The listing builds one solid part. Answer for the finished solid, in the listing's coordinates (mm). Face numbers are marked on the shaded views. Coordinates: 2 decimals unless noted, no trailing zeros. Answer in a Markdown table with one row per item.
```python
from build123d import *

# Parameters (mm, degrees)
F0_W      = 71.4375
F0_H      = 142.875
F1_DEPTH  = 6.35
F3_DEPTH  = 4.7625
F5_DEPTH  = 3.175
F6_R      = 3.175
F8_D      = 1.984375
F9_R      = 1.984375
F9_R_2    = 0.9921875
F10_DEPTH = 1.5875


with BuildPart() as f1:
    # F0 (on Top) → F1 (new body)
    with BuildSketch(Plane.XY):
        with BuildLine():
            Line((-40.084375, 71.4375), (-40.084375, 0))
            Line((-40.084375, 0), (-40.084375, -71.4375))
            ThreePointArc((-40.084375, -71.4375), (-39.1544390303, -73.6825640303), (-36.909375, -74.6125))
            Line((-36.909375, -74.6125), (36.909375, -74.6125))
            ThreePointArc((36.909375, -74.6125), (39.1544390303, -73.6825640303), (40.084375, -71.4375))
            Line((40.084375, -71.4375), (40.084375, 71.4375))
            ThreePointArc((40.084375, 71.4375), (39.1544390303, 73.6825640303), (36.909375, 74.6125))
            Line((36.909375, 74.6125), (-36.909375, 74.6125))
            ThreePointArc((-36.909375, 74.6125), (-39.1544390303, 73.6825640303), (-40.084375, 71.4375))
        make_face()
        with Locations((-1.190625, 0)):
            Rectangle(F0_W, F0_H, mode=Mode.SUBTRACT)
    extrude(amount=F1_DEPTH)

    # F2 (on face) → F3 (join)
    with BuildSketch(Plane(origin=(0, 0, 0), x_dir=(1, 0, 0), z_dir=(0, 0, -1))):
        with BuildLine():
            Line((-40.084375, 71.4375), (-40.084375, -71.4375))
            ThreePointArc((-40.084375, -71.4375), (-39.1544390303, -73.6825640303), (-36.909375, -74.6125))
            Line((-36.909375, -74.6125), (36.909375, -74.6125))
            ThreePointArc((36.909375, -74.6125), (39.1544390303, -73.6825640303), (40.084375, -71.4375))
            Line((40.084375, -71.4375), (40.084375, 71.4375))
            ThreePointArc((40.084375, 71.4375), (39.1544390303, 73.6825640303), (36.909375, 74.6125))
            Line((36.909375, 74.6125), (-36.909375, 74.6125))
            ThreePointArc((-36.909375, 74.6125), (-39.1544390303, 73.6825640303), (-40.084375, 71.4375))
        make_face()
        Polygon((-36.909375, -19.84375), (-36.909375, 71.4375), (34.528125, 71.4375), (34.528125, -19.84375), (34.528125, -71.4375), (-36.909375, -71.4375), align=None, mode=Mode.SUBTRACT)
        Polygon((34.528125, 71.4375), (-36.909375, 71.4375), (-36.909375, -19.84375), (-32.146875, -19.84375), (-32.146875, -14.2875), (-34.925, -14.2875), (-34.925, 15.08125), (-34.925, 24.60625), (-34.925, 66.675), (-32.146875, 66.675), (-32.146875, 69.453125), (29.765625, 69.453125), (29.765625, 66.675), (32.54375, 66.675), (32.54375, 24.60625), (32.54375, 15.08125), (32.54375, -14.2875), (29.765625, -14.2875), (29.765625, -19.84375), (34.528125, -19.84375), align=None)
        Polygon((-32.146875, -19.84375), (-36.909375, -19.84375), (-36.909375, -71.4375), (34.528125, -71.4375), (34.528125, -19.84375), (29.765625, -19.84375), (29.765625, -24.60625), (32.54375, -24.60625), (32.54375, -66.675), (29.765625, -66.675), (29.765625, -69.453125), (-32.146875, -69.453125), (-32.146875, -66.675), (-34.925, -66.675), (-34.925, -24.60625), (-32.146875, -24.60625), align=None)
    extrude(amount=-F3_DEPTH)

    # F4 (on face) → F5 (join)
    with BuildSketch(Plane(origin=(0, 0, 0), x_dir=(1, 0, 0), z_dir=(0, 0, -1))):
        with BuildLine():
            ThreePointArc((-36.909375, 74.6125), (-39.1544390303, 73.6825640303), (-40.084375, 71.4375))
            Line((-40.084375, 71.4375), (-40.084375, -71.4375))
            ThreePointArc((-40.084375, -71.4375), (-39.1544390303, -73.6825640303), (-36.909375, -74.6125))
            Line((-36.909375, -74.6125), (36.909375, -74.6125))
            ThreePointArc((36.909375, -74.6125), (39.1544390303, -73.6825640303), (40.084375, -71.4375))
            Line((40.084375, -71.4375), (40.084375, 71.4375))
            ThreePointArc((40.084375, 71.4375), (39.1544390303, 73.6825640303), (36.909375, 74.6125))
            Line((36.909375, 74.6125), (-36.909375, 74.6125))
        make_face()
        Polygon((29.765625, 66.675), (32.54375, 66.675), (32.54375, -14.2875), (29.765625, -14.2875), (29.765625, -24.60625), (32.54375, -24.60625), (32.54375, -66.675), (29.765625, -66.675), (29.765625, -69.453125), (-32.146875, -69.453125), (-32.146875, -66.675), (-34.925, -66.675), (-34.925, -24.60625), (-32.146875, -24.60625), (-32.146875, -14.2875), (-34.925, -14.2875), (-34.925, 66.675), (-32.146875, 66.675), (-32.146875, 69.453125), (29.765625, 69.453125), align=None, mode=Mode.SUBTRACT)
        Polygon((32.54375, -14.2875), (32.54375, 66.675), (29.765625, 66.675), (29.765625, 69.453125), (-32.146875, 69.453125), (-32.146875, 66.675), (-34.925, 66.675), (-34.925, -14.2875), (-32.146875, -14.2875), (-32.146875, -24.60625), (-34.925, -24.60625), (-34.925, -66.675), (-32.146875, -66.675), (-32.146875, -69.453125), (29.765625, -69.453125), (29.765625, -66.675), (32.54375, -66.675), (32.54375, -24.60625), (29.765625, -24.60625), (29.765625, -14.2875), align=None)
    extrude(amount=F5_DEPTH)

    # F6
    f6_edges = [f1.edges().sort_by_distance(p)[0] for p in [
        (-40.084375, 0, -3.175),
    ]]
    fillet(f6_edges, radius=F6_R)

    # F8 (through all)
    with Locations(Plane.XY.offset(4.7625)):
        with Locations((-34.13125, -68.659375), (31.75, -68.659375), (31.75, 68.659375), (-34.13125, 68.659375)):
            Hole(F8_D / 2)

    # F9 (on face) → F10 (cut)
    with BuildSketch(Plane(origin=(0, 0, -3.175), x_dir=(1, 0, 0), z_dir=(0, 0, -1))):
        with Locations((-34.13125, 68.659375)):
            Circle(F9_R)
        with Locations((-34.13125, 68.659375)):
            Circle(F9_R_2, mode=Mode.SUBTRACT)
        with Locations((31.75, 68.659375)):
            Circle(F9_R)
        with Locations((31.75, 68.659375)):
            Circle(F9_R_2, mode=Mode.SUBTRACT)
        with Locations((-34.13125, -68.659375)):
            Circle(F9_R)
        with Locations((-34.13125, -68.659375)):
            Circle(F9_R_2, mode=Mode.SUBTRACT)
        with Locations((31.75, -68.659375)):
            Circle(F9_R)
        with Locations((31.75, -68.659375)):
            Circle(F9_R_2, mode=Mode.SUBTRACT)
    extrude(amount=-F10_DEPTH, mode=Mode.SUBTRACT)


solid = f1.part
```
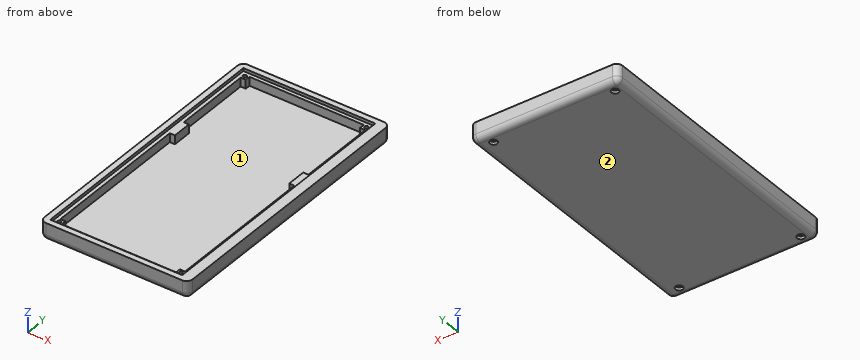
Item 1: A cutting plane is placed at C-C, the plane z = 3. Count the separate pieces of the cut face and the enclosed holes in it, plus the area to 3 significant figures.
Findings below:
| item | result |
|---|---|
| separate pieces | 1 |
| enclosed holes | 5 |
| area | 2,660 mm2 |
Item 2: Flat-ended cylindrical pins translate along their axes: pin 1 Ø3 at (x, z) = (-11, -2) entering from -Y; pin 2 Ø1.2 at (x, y) = (-34, 69.5) entering from -Z; pin 3 Ø1.8 at (x, y) = (-34.13, 68.66) entering from -Z; pin 4 Ø3 at (x, y) = (-34.13, -68.66) entering from +Z. Find the tip coordinate at first contact, or state that the pin passes through.
Findings below:
| item | result |
|---|---|
| pin 1 | stops at y = -74.57 |
| pin 2 | stops at z = -1.59 |
| pin 3 | passes through |
| pin 4 | stops at z = 4.76 |
Item 3: Determine the mould class of the marked faces 1 and 2 for opening direction X: +X half, -X half, draft (parallel to the pull), parting line (faces both ways), or undercut.
Findings below:
| item | result |
|---|---|
| face 1 | undercut |
| face 2 | draft |
Item 4: Find the intervals of material crossed by probe 1 along Y at (x, z) = (-33, 3.5) (1 decimal); probe 2 along Y at (x, z) = (31.75, 1.5) (1 decimal); probe 3 along Y at (x, z) = (-34, 2.25) (1 decimal), in increasing order.
Findings below:
| item | result |
|---|---|
| probe 1 | y = -74.6 to -66.7, 14.3 to 24.6, 66.7 to 74.6 |
| probe 2 | y = -74.6 to -69.7, -67.7 to -66.7, 14.3 to 24.6, 66.7 to 67.7, 69.7 to 74.6 |
| probe 3 | y = -74.6 to -69.6, -67.7 to -66.7, 14.3 to 24.6, 66.7 to 67.7, 69.6 to 74.6 |
